Verification items for the finished model (mm, model axes). Coordinates: 2 decimals unless noted, no trailing zeros. Write each loop counter-clockwise with the first axis right and the second up, starting at its lowest first coordinate (ties: lowest second). Pieces come first, ordered by that corner, then holes. Notation, with made-up numbers: (74.5, -36.5) - (83.5, -36.5) arc R31 ccw to (83.5, -12.5) - close; hole circle Ø9 at (-14, -10.75). An arc over 180 degrees is marked (long way). Use one line per item in the form item = value. Start each with the question number.
(1) Gauge pin test, flat end, axial feed: pin 1 Ø9 at (x, z) = (27.5, 15.5) entering from -Y. Record the tip position at first contact, or that the pin passes through.
(2) Sectioned sample at B-B (z = 25). Record the cut outline in (x, y), and give its area (3 significant figures).
(3) Sectioned sample at D-D (x = 28.5). Record the cut outline in (y, z), and give its area (3 significant figures).
(4) Material ranges on line 1 (Y direction, x = 38, z = 9.25); line 2 (X direction, y = 58, z = 27.5); line 3 (X direction, y = 3.5, z = 28.75), recorded low to high. Write a range as [from, to].
(5) Sectioned sample at C-C (z = 7). Record the cut outline in (x, y).
(6) Sectioned sample at A-A (x = 8). Record the cut outline in (y, z).
Autodesk Fusion 360 part; units mm, degrees
sketch "Esquisse1" plane through (0, 0, 0) normal (0, 0, 1) x (1, 0, 0)
  line L0 (0, 0) -> (58, 0)
  line L1 (58, 0) -> (58, 62)
  line L2 (58, 62) -> (0, 62)
  line L3 (0, 62) -> (0, 0)
  dimension "d1" = 58
  dimension "d2" = 62
extrude "Extrusion1" add sketch "Esquisse1" along normal blind 30
fillet "Congé1" radius 3 4 edges at (58, 31, 30) (58, 31, 0) (0, 31, 30) (0, 31, 0)
sketch "Esquisse2" plane through (0, 0, 0) normal (0, -1, 0) x (1, 0, 0)
  arc A0 (0, 3) -> (3, 0) centre (3, 3) ccw
  line L0 (3, 0) -> (55, 0)
  arc A1 (55, 0) -> (58, 3) centre (55, 3) ccw
  line L1 (58, 3) -> (58, 27)
  arc A2 (58, 27) -> (55, 30) centre (55, 27) ccw
  line L2 (55, 30) -> (3, 30)
  arc A3 (3, 30) -> (0, 27) centre (3, 27) ccw
  line L3 (0, 27) -> (0, 3)
  circle A4 centre (8, 24) radius 3
  dimension "d7" = 6
  dimension "d8" = 6
  dimension "d9" = 8
sketch "Esquisse3" plane through (0, 0, 0) normal (0, -1, 0) x (1, 0, 0)
  line L0 (18.832, 28.0784) -> (16.384, 24.1616)
  line L1 (16.384, 24.1616) -> (18.552, 20.0833)
  line L2 (18.552, 20.0833) -> (23.168, 19.9216)
  line L3 (23.168, 19.9216) -> (25.616, 23.8384)
  line L4 (25.616, 23.8384) -> (23.448, 27.9167)
  line L5 (23.448, 27.9167) -> (18.832, 28.0784)
  line L6 (55, 30) -> (3, 30)
  line L7 (0, 27) -> (0, 3)
  point P0 (21, 24)
  dimension "d10" = 8
  dimension "d11" = 6
  dimension "d12" = 21
extrude "Extrusion2" add sketch "Esquisse2" sketch "Esquisse3" along normal blind 2 contours A4 of sketch 2
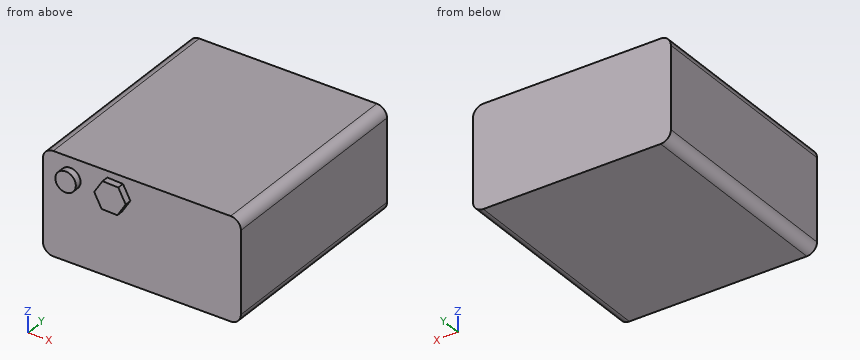
Answers below:
q1.pin_1 = 0
q2.outline = (0, 0) - (5.17, 0) - (5.17, -2) - (10.83, -2) - (10.83, 0) - (16.91, 0) - (16.91, -2) - (25, -2) - (25, 0) - (58, 0) - (58, 62) - (0, 62) - close
q2.area = 3,620 mm2
q3.outline = (0, 0) - (62, 0) - (62, 30) - (0, 30) - close
q3.area = 1,860 mm2
q4.line_1 = [0, 62]
q4.line_2 = [0.04, 57.96]
q4.line_3 = [0.56, 57.44]
q5.outline = (0, 0) - (58, 0) - (58, 62) - (0, 62) - close
q6.outline = (-2, 21) - (0, 21) - (0, 0) - (62, 0) - (62, 30) - (0, 30) - (0, 27) - (-2, 27) - close
